Here's how the part is built. I have some questions about the finished solid (model axes, mm). A direction names the side the tool comes from. Round coordinates to 2 decimals unless told otherwise and drop trailing zeros. Loops run counter-clockwise (first coordinate to the right, second up) from the corner with the lowest first, then second, coordinate; pieces in that order, holes last. Notation, with made-up numbers: M 38.5,57.25 L 64.5,57.25 A26 cw 64.5,87.25 Z; hole C 63,79 d9. An arc over 180 degrees is marked long. Use a Markdown table: item, result.
Autodesk Inventor part; units mm, degrees
ref_plane "Work Plane1" through (-7, -38, 0) normal (1, 0, 0) x (0, 1, 0)
ref_plane "XZ Plane" through (0, 0, 0) normal (0, 1, 0) x (-1, 0, 0)
ref_plane "XY Plane" through (0, 0, 0) normal (0, 0, 1) x (1, 0, 0)
sketch "Sketch1" plane through (0, 0, 0) normal (0, 0, 1) x (1, 0, 0)
  line L0 (0, 75) -> (0, -75)
  line L1 (7, 75) -> (0, 75)
  line L2 (7, -75) -> (0, -75)
  line L3 (7, -75) -> (7, 75)
  line L4 (7, 1) -> (8, 1)
  line L5 (8, 1) -> (8, -1)
  line L6 (8, -1) -> (7, -1)
  point P0 (0, 0)
  point P1 (0, 0)
  point P2 (3.5, 75)
  point P3 (8, 0)
  dimension "d17" = 14
  dimension "d42" = 150
  dimension "d43" = 75
  dimension "d44" = 2
  dimension "d45" = 16
revolve "Revolution1" add sketch "Sketch1" angle 360 about axis through (0, 75, 0) along (0, -1, 0)
sketch "Sketch4" plane through (0, 75, 0) normal (0, 1, 0) x (1, 0, 0)
  point P0 (0, 0)
  point P1 (0, 0)
hole "Hole1" at (0, 75, 0) direction (0, -1, 0) diameter 6.647 depth 22.2 tip angle 118
chamfer "Chamfer1" distance 1 angle 45 1 edges at (-7, 75, 0)
ref_plane "Work Plane1" through (-7, -38, 0) normal (1, 0, 0) x (0, 1, 0)
sketch "Sketch5" plane through (-7, -38, 0) normal (1, 0, 0) x (0, 1, 0)
  line L0 (-37, 7) -> (-37, -7)
  line L1 (112, -7) -> (112, 7)
  line L2 (98, 0) -> (83, 0) construction
  line L3 (98, -2.5) -> (83, -2.5)
  line L4 (83, 2.5) -> (98, 2.5)
  arc A0 (98, -2.5) -> (98, 2.5) centre (98, 0) ccw
  arc A1 (83, 2.5) -> (83, -2.5) centre (83, 0) ccw
  line L5 (113, 6) -> (113, -6)
  line L6 (63, 0) -> (48, 0) construction
  line L7 (63, -2.5) -> (48, -2.5)
  line L8 (48, 2.5) -> (63, 2.5)
  arc A2 (63, -2.5) -> (63, 2.5) centre (63, 0) ccw
  arc A3 (48, 2.5) -> (48, -2.5) centre (48, 0) ccw
  point P0 (38, 0)
  point P1 (90.5, 0)
  point P2 (55.5, 0)
  dimension "d36" = 5
  dimension "d37" = 15
  dimension "d39" = 15
  dimension "d46" = 5
  dimension "d47" = 15
  dimension "d48" = 35
extrude "Extrusion3" cut sketch "Sketch5" along normal blind 3
equation "\"d47\" = d37"
properties part number "приводной вал"
Q1. For faces 1 (the cylindrical face through (1.27, 63.74, 3.07)), 2 (the flat face through (0, -75, 0)), 3 (the flat face through (-5, 52, 2.5)), which set-ups out of +Z, -Z, +X, -X, +Y, -Y let a thin tool reach every point of the face, with its end or its side?
Return value:
| item | result |
|---|---|
| face 1 | +Y |
| face 2 | +Z, -Z, +X, -X, -Y |
| face 3 | -X |
Q2. Will these pins go through, and if not, where does the flat tip stop? P1, Ø5.5, axis at y = 13, z = 0.5, coming from the -X side; P2, Ø2, axis at y = -48.5, z = -2, coming from the +X side; P3, Ø8, axis at x = 4.5, y = -21, coming from the -Z side.
Return value:
| item | result |
|---|---|
| P1 | stops at x = -6.54 |
| P2 | stops at x = 6.93 |
| P3 | stops at z = -6.98 |
Q3. We'd pull the mould along Y, two halves only. Please class faces 4 (the cylindrical face through (-5.5, 42.5, -0.1)), 5 (the flat face through (3, 75, -3)), 6 (the flat face through (4, -1, -6)): pulls with the +Y half, pulls with the -Y half, needs draft (parallel to the pull), parting line crosses it, or undercut.
Return value:
| item | result |
|---|---|
| face 4 | undercut |
| face 5 | pulls with the +Y half |
| face 6 | pulls with the -Y half |
Q4. Imagine slicing it at A-A, the plane y = -9. Please give me the cut outline in (x, z), then the cut area to 3 significant figures.
Return value:
| item | result |
|---|---|
| outline | C 0,0 d14 |
| area | 154 mm^2 |
Q5. I need wall thicknesses on line 1 (X direction, y = 69.25, z = 0); line 2 (X direction, y = 59, z = 0). Which ranges of each line are inside material? Lowest first, please. Write a range as from..to.
Return value:
| item | result |
|---|---|
| line 1 | x = -7..-3.32, 3.32..7 |
| line 2 | x = -4..-3.32, 3.32..7 |
